Could you check a few things on this drawing? It's one solid part, dimensions in mm from its lowest x, y, z. A direction names the side the tool comes from. Give positions to 0.01 mm unless a question says otherwise; leave off trailing zeros. Order: outer loops, then holes, each group sorted by start corner. A loop starts at its lowest first (then second) coordinate and runs counter-clockwise, first axis right, second up. Notation, with made-up numbers: (3, 34) - (45, 34) arc R16 ccw to (45, 47) - close; hole circle Ø9 at (-1, -17). An arc over 180 degrees is marked (long way). Put each result on its own line as item: value.
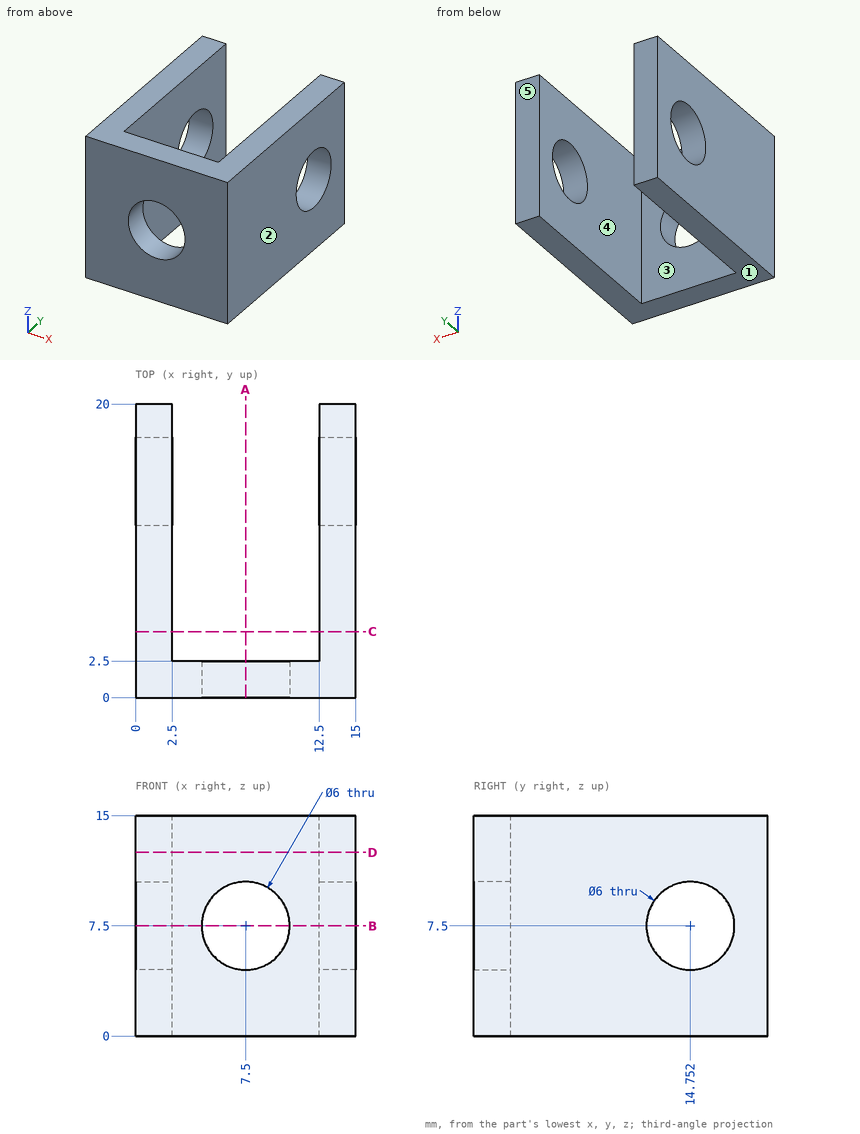
1) Suppose I cut it at D-D, the plane z = 12.5. List the corners of the cut face in (x, y) for me, and give its area (3 significant figures).
Filled in:
outline: (0, 0) - (15, 0) - (15, 20) - (12.5, 20) - (12.5, 2.5) - (2.5, 2.5) - (2.5, 20) - (0, 20) - close
area: 125 mm^2
2) Suppose I cut it at A-A, the plane x = 7.5. List the corners of the cut face in (y, z) for me, and give its area (3 significant figures).
Filled in:
outline: (0, 0) - (2.5, 0) - (2.5, 4.5) - (0, 4.5) - close; (0, 10.5) - (2.5, 10.5) - (2.5, 15) - (0, 15) - close
area: 22.5 mm^2
3) Which directions (+Z, -Z, +X, -X, +Y, -Y) give clear straight access to the entire face, cutting with the end or side of a thin tool? Please do the marked faces 4 and 5.
Filled in:
face 4: +Z, -Z, +Y
face 5: +Z, -Z, +X, -X, +Y
4) Suppose I cut it at C-C, the plane y = 4.5. List the corners of the cut face in (x, z) for me, and give its area (3 significant figures).
Filled in:
outline: (0, 0) - (2.5, 0) - (2.5, 15) - (0, 15) - close; (12.5, 0) - (15, 0) - (15, 15) - (12.5, 15) - close
area: 75.0 mm^2
5) If I drill on line 1 (X direction, y = 0.55, z = 7.5); line 2 (X direction, y = 11.5, z = 6.5); line 3 (Y direction, x = 0.9, z = 7.5), over which ranges is the centre line in solid material (lowest first)? Write a range as [from, to].
Filled in:
line 1: x = [0, 4.5], [10.5, 15]
line 2: x = [0, 2.5], [12.5, 15]
line 3: y = [0, 11.75], [17.75, 20]
6) We'd pull the mould along X, two halves only. Please class the marked faces 1, 2 and 3: pulls with the +X half, pulls with the -X half, needs draft (parallel to the pull), parting line crosses it, or undercut.
Filled in:
face 1: needs draft
face 2: pulls with the +X half
face 3: undercut
7) Suppose I cut it at B-B, the plane z = 7.5. List the corners of the cut face in (x, y) for me.
Filled in:
outline: (0, 0) - (4.5, 0) - (4.5, 2.5) - (2.5, 2.5) - (2.5, 11.75) - (0, 11.75) - close; (0, 17.75) - (2.5, 17.75) - (2.5, 20) - (0, 20) - close; (10.5, 0) - (15, 0) - (15, 11.75) - (12.5, 11.75) - (12.5, 2.5) - (10.5, 2.5) - close; (12.5, 17.75) - (15, 17.75) - (15, 20) - (12.5, 20) - close
